Could you check a few things on this model? Use its own coordinates, in mm. A direction names the side the tool comes from. Give positions to 0.01 mm unless a question says otherwise; leave off trailing zeros. Write each loop counter-clockwise with the first axis right and the second up, starting at its lowest first coordinate (ties: lowest second). Pieces come first, ordered by that corner, then holes. Notation, with made-up numbers: (24, 6) - (59, 6) arc R14 ccw to (59, 22) - close; hole circle Ø3 at (23, -38.5). An arc over 180 degrees is marked (long way). Answer as CSV lines item,"result". Start each with the question number.
Q1. Imagine slicing it at D-D on y = -1.5. List the corners of the cut face in (x, z) for me.
Q2. Imagine slicing it at A-A on z = -21.15. List the corners of the cut face in (x, y) for me, and give its area (3 significant figures).
Q3. We'd pull the mould along X, two halves only. Please class faces 4 (the face through (7, 0, -62.3)), 5 (the face through (2.25, 0.06, -61.73)), 6 (the face through (-27.75, 1.97, -36.73)): pulls with the +X half, pulls with the -X half, needs draft (parallel to the pull), parting line crosses it, or undercut.
Q4. Imagine slicing it at C-C on z = -5.65. List the corners of the cut face in (x, y) for me.
Q5. If I drill on line 1 along X through (y, z) = (1.45, -36.65); line 2 along Z through (x, y) = (-26, 2.35), over which ranges is the centre line in solid material (lowest first)?
Q6. On a 3-axis mill with a long thin cutter (end or side, diameter ignored), from which of +Z, -Z, +X, -X, +Y, -Y can I reach the whole of each face in a straight line? I mean faces 1 (the face through (4, -2, -42.3)), 2 (the face through (10.15, 2.03, -1.43)), 3 (the face through (-15, 2, -42.3)). Say none if no direction works.
Q7. Imagine slicing it at B-B on x = -20. List the corners of the cut face in (y, z) for me.
Q8. Will these pins go through, and if not, where does the flat tip stop? pin 1 Ø2 at (x, z) = (5, -36.65) entering from -Y; pin 2 Ø1.2 at (x, y) = (7, -2) entering from +Z; pin 3 Ø2 at (x, y) = (-11.5, 3) entering from -Z; pin 4 Ø4.5 at (x, z) = (-26, -36.65) entering from +Y.
```python
from build123d import *

# Parameters (mm, degrees)
SKETCH2_R           = 1.75
SKETCH2_R_2         = 12.5
SKETCH2_R_3         = 1.85
BOSS_EXTRUDE1_DEPTH = 4
FILLET1_R           = 5
FILLET8_R           = 5
SKETCH5_R           = 1.85
BOSS_EXTRUDE2_DEPTH = 4
FILLET10_R          = 2


with BuildPart() as part:
    # Sketch2 → Boss-Extrude1 (new body)
    with BuildSketch(Plane(origin=(0, 0, 0), x_dir=(1, 0, 0), z_dir=(0, 1, 0))):
        Polygon((-30.65, 0), (-30.65, 42.3), (1.65, 42.3), (1.65, 62.3), (11.65, 62.3), (11.65, 42.3), (11.65, 0), align=None)
        with Locations((5, 5.65)):
            Circle(SKETCH2_R, mode=Mode.SUBTRACT)
        with Locations((5, 36.65)):
            Circle(SKETCH2_R, mode=Mode.SUBTRACT)
        with Locations((-26, 5.65)):
            Circle(SKETCH2_R, mode=Mode.SUBTRACT)
        with Locations((-26, 36.65)):
            Circle(SKETCH2_R, mode=Mode.SUBTRACT)
        with Locations((-9.5, 21.15)):
            Circle(SKETCH2_R_2, mode=Mode.SUBTRACT)
        with Locations((6.65, 56.8)):
            Circle(SKETCH2_R_3, mode=Mode.SUBTRACT)
        with Locations((6.65, 47.3)):
            Circle(SKETCH2_R_3, mode=Mode.SUBTRACT)
    extrude(amount=BOSS_EXTRUDE1_DEPTH)

    # Fillet1
    fillet1_edges = [part.edges().sort_by_distance(p)[0] for p in [
        (11.65, 2, 0),
        (-30.65, 2, 0),
        (-30.65, 2, -42.3),
    ]]
    fillet(fillet1_edges, radius=FILLET1_R)

    # Fillet8
    fillet8_edges = [part.edges().sort_by_distance(p)[0] for p in [
        (1.65, 2, -42.3),
    ]]
    fillet(fillet8_edges, radius=FILLET8_R)

    # Sketch5 → Boss-Extrude2 (add)
    with BuildSketch(Plane.XZ):
        with BuildLine():
            Line((11.65, -62.3), (1.65, -62.3))
            Line((1.65, -62.3), (1.65, -47.3))
            ThreePointArc((1.65, -47.3), (0.185533906, -43.764466094), (-3.35, -42.3))
            Line((-3.35, -42.3), (11.65, -42.3))
            Line((11.65, -42.3), (11.65, -62.3))
        make_face()
        with Locations((6.65, -47.3)):
            Circle(SKETCH5_R, mode=Mode.SUBTRACT)
        with Locations((6.65, -56.8)):
            Circle(SKETCH5_R, mode=Mode.SUBTRACT)
    extrude(amount=BOSS_EXTRUDE2_DEPTH)

    # Fillet10
    fillet10_edges = [part.edges().sort_by_distance(p)[0] for p in [
        (1.65, 0, -62.3),
        (11.65, 0, -62.3),
    ]]
    fillet(fillet10_edges, radius=FILLET10_R)


solid = part.part
```
Conclusion:
1,outline,"(-3.35, -42.3) arc R5 cw to (1.65, -47.3) - (1.65, -60.3) arc R2 ccw to (3.65, -62.3) - (9.65, -62.3) arc R2 ccw to (11.65, -60.3) - (11.65, -42.3) - close; hole circle Ø3.7 at (6.65, -56.8); hole circle Ø3.7 at (6.65, -47.3)"
2,outline,"(-30.65, 0) - (-22, 0) - (-22, 4) - (-30.65, 4) - close; (3, 0) - (11.65, 0) - (11.65, 4) - (3, 4) - close"
2,area,"69.2 mm^2"
3,face 4,"needs draft"
3,face 5,"pulls with the -X half"
3,face 6,"undercut"
4,outline,"(-30.65, 0) - (-27.75, 0) - (-27.75, 4) - (-30.65, 4) - close; (-24.25, 0) - (3.25, 0) - (3.25, 4) - (-24.25, 4) - close; (6.75, 0) - (11.65, 0) - (11.65, 4) - (6.75, 4) - close"
5,line 1,"-30.65 to -27.75, -24.25 to 3.25, 6.75 to 11.65"
5,line 2,"-42.29 to -38.4, -34.9 to -7.4, -3.9 to -0.01"
6,face 1,"+Z, +X, -X, -Y"
6,face 2,"+Z, +X, +Y, -Y"
6,face 3,"-Z, -X, +Y, -Y"
7,outline,"(0, -42.3) - (4, -42.3) - (4, -27.93) - (0, -27.93) - close; (0, -14.37) - (4, -14.37) - (4, 0) - (0, 0) - close"
8,pin 1,"through"
8,pin 2,"z = -42.3"
8,pin 3,"z = -42.3"
8,pin 4,"y = 4"
